Design review of the part built by this model. Coordinates are the model's own, in mm. A direction names the side the tool comes from. Coordinates: 2 decimals unless noted, no trailing zeros.
```python
from build123d import *

# Parameters (mm, degrees)
EXTRUDE1_DEPTH     = 17.78
SKETCH4_R          = 3.175
SKETCH4_R_2        = 3.175000002
CUT_EXTRUDE1_DEPTH = 17.78
SKETCH6_R          = 1.5875
SKETCH6_R_2        = 2.777849083
CUT_EXTRUDE3_DEPTH = 17.78
SKETCH5_W          = 17.78
SKETCH5_H          = 63.50740041
SKETCH5_H_2        = 63.507400408
CUT_EXTRUDE2_DEPTH = 5.08
SKETCH7_R          = 3.302
CUT_EXTRUDE4_DEPTH = 5.08
SKETCH9_R          = 3.175
CUT_EXTRUDE5_DEPTH = 17.78


with BuildPart() as part:
    # Sketch3 → Extrude1 (new body)
    with BuildSketch(Plane.XY):
        Polygon((10806.641666666, -6342.0625), (11340.041666666, -6342.0625), (11340.041666666, -5818.736838581), (11308.291666667, -5818.736838581), (11308.291666667, -5742.536838581), (10838.391666667, -5742.536838581), (10838.391666667, -5818.736838581), (10806.641666666, -5818.736838581), align=None)
    extrude(amount=-EXTRUDE1_DEPTH)

    # Sketch4 → Cut-Extrude1 (cut)
    with BuildSketch(Plane.XY):
        with Locations((11310.536730697, -5816.491774551)):
            Circle(SKETCH4_R)
        with Locations((10836.146602637, -5816.491774551)):
            Circle(SKETCH4_R_2)
    extrude(amount=-CUT_EXTRUDE1_DEPTH, mode=Mode.SUBTRACT)

    # Sketch6 → Cut-Extrude3 (cut)
    with BuildSketch(Plane.XY):
        with Locations((10851.409166666, -6294.4375)):
            Circle(SKETCH6_R)
        with Locations((10908.241666666, -6326.8225)):
            Circle(SKETCH6_R)
        with Locations((11073.341666666, -6326.8225)):
            Circle(SKETCH6_R)
        with Locations((11238.441666666, -6326.8225)):
            Circle(SKETCH6_R)
        with Locations((11295.274166666, -6294.4375)):
            Circle(SKETCH6_R)
        with Locations((11295.274166666, -6237.2875)):
            Circle(SKETCH6_R)
        with Locations((11263.841666666, -6220.099669291)):
            Circle(SKETCH6_R)
        with Locations((11295.274166666, -6180.1375)):
            Circle(SKETCH6_R)
        with Locations((11263.841666666, -6042.299669291)):
            Circle(SKETCH6_R)
        with Locations((11263.841666666, -5864.499669291)):
            Circle(SKETCH6_R)
        with Locations((11299.401666666, -5793.344238991)):
            Circle(SKETCH6_R)
        with Locations((11299.401666666, -5755.236838581)):
            Circle(SKETCH6_R)
        with Locations((10847.281666666, -5755.236838581)):
            Circle(SKETCH6_R)
        with Locations((10847.281666666, -5793.344238991)):
            Circle(SKETCH6_R)
        with Locations((10882.841666666, -6042.299669291)):
            Circle(SKETCH6_R_2)
        with Locations((10851.409166666, -6180.1375)):
            Circle(SKETCH6_R)
        with Locations((10882.841666666, -6220.099669291)):
            Circle(SKETCH6_R)
        with Locations((10851.409166666, -6237.2875)):
            Circle(SKETCH6_R)
        with Locations((10882.841666666, -5864.499669291)):
            Circle(SKETCH6_R)
    extrude(amount=-CUT_EXTRUDE3_DEPTH, mode=Mode.SUBTRACT)

    # Sketch5 → Cut-Extrude2 (cut)
    with BuildSketch(Plane.XY):
        Polygon((11073.341666666, -6317.9325), (10806.641666666, -6317.9325), (10806.641666666, -6335.7125), (11340.041666666, -6335.7125), (11340.041666666, -6317.9325), align=None)
        with Locations((10847.281666667, -5774.290538786)):
            Rectangle(SKETCH5_W, SKETCH5_H)
        with Locations((11299.401666667, -5774.290538785)):
            Rectangle(SKETCH5_W, SKETCH5_H_2)
    extrude(amount=-CUT_EXTRUDE2_DEPTH, mode=Mode.SUBTRACT)

    # Sketch7 → Cut-Extrude4 (cut)
    with BuildSketch(Plane.XY):
        with Locations((10853.926602637, -5803.79917496)):
            Circle(SKETCH7_R)
        with Locations((11292.756730697, -5803.799174959)):
            Circle(SKETCH7_R)
    extrude(amount=-CUT_EXTRUDE4_DEPTH, mode=Mode.SUBTRACT)

    # Sketch9 → Cut-Extrude5 (cut)
    with BuildSketch(Plane.XY):
        with Locations((10879.616654067, -5760.644320781)):
            Circle(SKETCH9_R)
        with Locations((10936.816666667, -5760.644320781)):
            Circle(SKETCH9_R)
        with Locations((11209.816654067, -5760.644320781)):
            Circle(SKETCH9_R)
        with Locations((11267.016666667, -5760.644320781)):
            Circle(SKETCH9_R)
    extrude(amount=-CUT_EXTRUDE5_DEPTH, mode=Mode.SUBTRACT)


solid = part.part
```
(1) Consider section A-A (z = -14.25). State how many separate pieces and enclosed holes the cut face has, plus the area to 3 significant figures.
(2) Mouldability with a two-part tool opening along Y and no side actions: class faces 1 (the flat face through (11077, -5742.537, -9)), 2 (the flat face through (10806.642, -6077, -9)), 3 (the flat face through (11070, -6342.062, -9)), 4 (the flat face through (11070, -6327, -5.08)) as +Y half, -Y half, draft (parallel to the pull), parting line (faces both ways), or undercut.
(3) For faces 5 (the flat face through (11327, -5818.737, -9)), 6 (the flat face through (10820, -5818.737, -9)), 7 (the flat face through (11070, -6038, -17.78)), list the 3-axis set-ups (+Z, -Z, +X, -X, +Y, -Y) from which the entire face can be reached by the end or side of a thin tool; tool diameter is ignored.
(4) Insertion check: pin 1 Ø9 at (y, z) = (-5774.5, -10.5) entering from +X; pin 2 Ø3 at (x, y) = (10847.28, -5793.34) entering from -Z; pin 3 Ø4 at (x, z) = (10847, -2.5) entering from +Y; pin 4 Ø9 at (y, z) = (-5789.5, -10) entering from -X. Each pin has a flat end and moves straight along its axis. Give the tip position at first contact, or say it passes through.
(5) Wall thickness on line 1 (X direction, y = -5793.5, z = -15.75); line 2 (X direction, y = -6295, z = -11.75); line 3 (Y direction, x = 10844, z = -3): over which ranges is each line inside the solid? List them lowest first.
Results:
1. separate pieces: 1
1. enclosed holes: 23
1. area: 315,000 mm2
2. face 1: +Y half
2. face 2: draft
2. face 3: -Y half
2. face 4: undercut
3. face 5: +Z, -Z, +X, +Y
3. face 6: +Z, -Z, -X, +Y
3. face 7: -Z, +X, -X, +Y, -Y
4. pin 1: stops at x = 11308.29
4. pin 2: passes through
4. pin 3: stops at y = -5806.04
4. pin 4: stops at x = 10838.39
5. line 1: x = 10838.39 to 10845.7, 10848.86 to 11297.82, 11300.98 to 11308.29
5. line 2: x = 10806.64 to 10849.92, 10852.89 to 11293.79, 11296.76 to 11340.04
5. line 3: y = -6342.06 to -6335.71, -6317.93 to -5806.04
